The model under review builds one solid part; all positions refer to its coordinate system, in mm. Face numbers are marked on the shaded views. Give positions to 0.01 mm unless a question says otherwise; leave off trailing zeros. Order: outer loops, then holes, each group sorted by start corner. A loop starts at its lowest first (then second) coordinate and runs counter-clockwise, first axis right, second up.
```python
from build123d import *


with BuildPart() as f1:
    # F0 (on Front) → F1 (revolve)
    with BuildSketch(Plane.XZ):
        with BuildLine():
            Line((0, 59.608808), (0, 53))
            Line((0, 53), (1.98564, 53))
            ThreePointArc((1.98564, 53), (2.243281, 52.893281), (2.35, 52.63564))
            Line((2.35, 52.63564), (2.35, 0))
            Line((2.35, 0), (4.6, 0))
            Line((4.6, 0), (4.6, 52.208291))
            ThreePointArc((4.6, 52.208291), (4.534388, 52.611216), (4.344333, 52.972509))
            ThreePointArc((4.344333, 52.972509), (2.062526, 56.218884), (0, 59.608808))
        make_face()
        with BuildLine():
            ThreePointArc((-10, 89.123821), (-7.453856, 70.38262), (0, 53))
            Line((0, 53), (0, 59.608808))
            ThreePointArc((0, 59.608808), (-5.780208, 73.866049), (-7.75, 89.123821))
            Line((-7.75, 89.123821), (-10, 89.123821))
        make_face()
        with BuildLine():
            ThreePointArc((-9.257581, 102.835982), (-9.814259, 95.989943), (-10, 89.123821))
            Line((-10, 89.123821), (-7.75, 89.123821))
            ThreePointArc((-7.75, 89.123821), (-7.56755, 95.8683), (-7.020734, 102.59305))
            Line((-7.020734, 102.59305), (0, 167.237922))
            Line((0, 167.237922), (0, 188.077089))
            Line((0, 188.077089), (-9.257581, 102.835982))
        make_face()
        with BuildLine():
            Line((0, 188.077089), (0, 167.237922))
            Line((0, 167.237922), (69.104384, 803.530977))
            ThreePointArc((69.104384, 803.530977), (69.349117, 804.008226), (69.85, 804.2))
            Line((69.85, 804.2), (69.85, 806.45))
            ThreePointArc((69.85, 806.45), (67.846469, 805.682905), (66.867537, 803.773909))
            Line((66.867537, 803.773909), (0, 188.077089))
        make_face()
    revolve(axis=Axis((69.85, 0, 403.225), (0, 0, 1)))


solid = f1.part
```
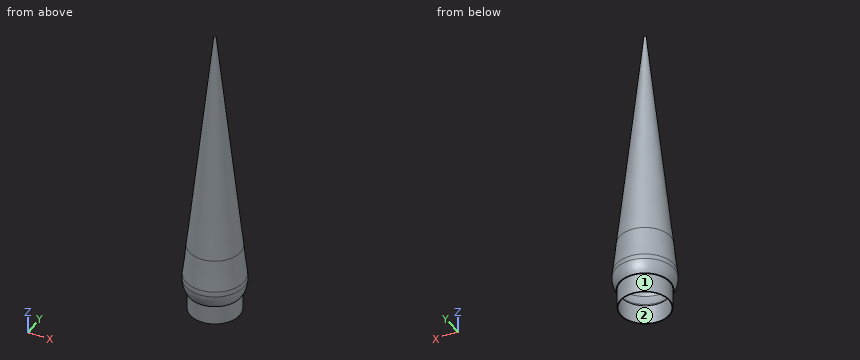
Item 1: Draft analysis for pull direction Y (two halves, no side actions). For the marked faces 1 and 2, state which applies: released by +Y, released by -Y, zero draft, split by the parting line, or undercut.
Values found:
face 1: split by the parting line
face 2: undercut
Item 2: Take a section at A-A (z = 625). Give the boundary of the cut face in (x, y).
Values found:
outline: circle Ø44.8 at (69.85, 0); hole circle Ø40.27 at (69.85, 0)
Item 3: Clearance check with flat-ended pins moving along their axes: pin 1 Ø2 at (x, z) = (14, 229.5) entering from +Y; pin 2 Ø12 at (x, z) = (63.5, 622) entering from +Y; pin 3 Ø12 at (y, z) = (-10, 697) entering from -X. State where each tip first meets the part, or that it passes through.
Values found:
pin 1: stops at y = 35.54
pin 2: stops at y = 23.09
pin 3: stops at x = 55.71
Item 4: For line 1 (Y direction, x = 69.85, z = 21.5); line 2 (X direction, y = 0, z = 42.5); line 3 (X direction, y = 9, z = 212), list the stretches that pass through material, from the lowest coordinate up.
Values found:
line 1: y = -67.5 to -65.25, 65.25 to 67.5
line 2: x = 2.35 to 4.6, 135.1 to 137.35
line 3: x = 3.2 to 5.49, 134.21 to 136.5
Item 5: Take a section at B-B (z = 301.5). Give the boundary of the cut face in (x, y).
Values found:
outline: circle Ø115.06 at (69.85, 0); hole circle Ø110.54 at (69.85, 0)
